For this review, take the finished solid that the model builds, in its own axes (mm). Give positions to 0.01 mm unless a question says otherwise; leave off trailing zeros. Order: outer loops, then holes, each group sorted by start corner. A loop starts at its lowest first (then second) coordinate and runs counter-clockwise, first axis right, second up. Notation, with made-up numbers: (24, -7) -> (39, -7) arc R31 cw to (39, 17) -> close; hole circle Ø2 at (-0.5, 40). An arc over 180 degrees is marked (long way). Return JSON: item names as keys, results as strings. Group by question number.
1) Add section D-D (z = -6). Give the boundary of the cut face in (x, y).
2) Insertion check: P1, Ø0.7, axis at x = 27, y = 2, coming from the -Z side; P2, Ø1.5, axis at y = 2, z = -51.5, coming from the -X side; P3, Ø2.5, axis at x = 14, z = -5.2, coming from the -Y side. Each pin has a flat end and moves straight along its axis. Give the tip position at first contact, or say it passes through.
3) To check wall thickness, follow line 1 along X through (y, z) = (1.45, -36.2); line 2 along Z through (x, y) = (14, 2.05); line 3 along Z through (x, y) = (54.1, 1.15). State the ranges of each line that lie inside material, in increasing order.
4) Add section C-C (x = 45). Give the boundary of the cut face in (y, z), then the cut area to 3 significant figures.
5) Add section B-B (z = -42). Give the boundary of the cut face in (x, y), then the cut area to 3 significant figures.
6) Add section A-A (x = 29.5). Give the boundary of the cut face in (y, z).
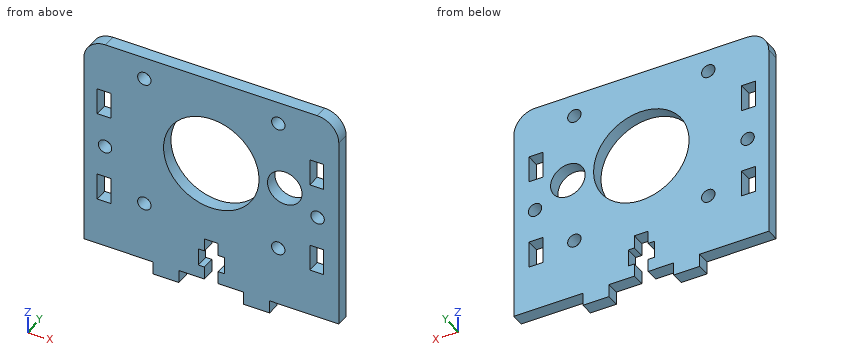
from build123d import *

# Parameters (mm, degrees)
CROQUIS1_R              = 1.55
CROQUIS1_R_2            = 11.05
CROQUIS1_R_3            = 4
CROQUIS1_W              = 3.2
CROQUIS1_H              = 6.2
SALIENTE_EXTRUIR1_DEPTH = 3


with BuildPart() as part:
    # Croquis1 → Saliente-Extruir1 (new body)
    with BuildSketch(Plane(origin=(0, 0, 0), x_dir=(1, 0, 0), z_dir=(0, 1, 0))):
        with BuildLine():
            Line((5, 0), (54, 0))
            ThreePointArc((54, 0), (57.535533906, 1.464466094), (59, 5))
            Line((59, 5), (59, 50))
            Line((59, 50), (43, 50))
            Line((43, 50), (43, 53))
            Line((43, 53), (37, 53))
            Line((37, 53), (37, 50))
            Line((37, 50), (31.1, 50))
            Line((31.1, 50), (31.1, 47))
            Line((31.1, 47), (32.5, 47))
            Line((32.5, 47), (32.5, 43))
            Line((32.5, 43), (31.1, 43))
            Line((31.1, 43), (31.1, 40))
            Line((31.1, 40), (27.9, 40))
            Line((27.9, 40), (27.9, 43))
            Line((27.9, 43), (26.5, 43))
            Line((26.5, 43), (26.5, 47))
            Line((26.5, 47), (27.9, 47))
            Line((27.9, 47), (27.9, 50))
            Line((27.9, 50), (22, 50))
            Line((22, 50), (22, 53))
            Line((22, 53), (16, 53))
            Line((16, 53), (16, 50))
            Line((16, 50), (0, 50))
            Line((0, 50), (0, 5))
            ThreePointArc((0, 5), (1.464466094, 1.464466094), (5, 0))
        make_face()
        with Locations((4.9, 25.3)):
            Circle(CROQUIS1_R, mode=Mode.SUBTRACT)
        with Locations((29.5, 20.7)):
            Circle(CROQUIS1_R_2, mode=Mode.SUBTRACT)
        with Locations((14, 36.2)):
            Circle(CROQUIS1_R, mode=Mode.SUBTRACT)
        with Locations((45, 36.2)):
            Circle(CROQUIS1_R, mode=Mode.SUBTRACT)
        with Locations((45, 5.2)):
            Circle(CROQUIS1_R, mode=Mode.SUBTRACT)
        with Locations((14, 5.2)):
            Circle(CROQUIS1_R, mode=Mode.SUBTRACT)
        with Locations((46.5, 20.7)):
            Circle(CROQUIS1_R_3, mode=Mode.SUBTRACT)
        with Locations((54.1, 25.3)):
            Circle(CROQUIS1_R, mode=Mode.SUBTRACT)
        with Locations((4.7, 14.7)):
            Rectangle(CROQUIS1_W, CROQUIS1_H, mode=Mode.SUBTRACT)
        with Locations((4.7, 35.9)):
            Rectangle(CROQUIS1_W, CROQUIS1_H, mode=Mode.SUBTRACT)
        with Locations((53.9, 35.9)):
            Rectangle(CROQUIS1_W, CROQUIS1_H, mode=Mode.SUBTRACT)
        with Locations((53.9, 14.7)):
            Rectangle(CROQUIS1_W, CROQUIS1_H, mode=Mode.SUBTRACT)
    extrude(amount=SALIENTE_EXTRUIR1_DEPTH)


solid = part.part
Evaluation:
{
 "1": {"outline": "(0, 0) -> (12.67, 0) -> (12.67, 3) -> (0, 3) -> close; (15.33, 0) -> (43.67, 0) -> (43.67, 3) -> (15.33, 3) -> close; (46.33, 0) -> (59, 0) -> (59, 3) -> (46.33, 3) -> close"},
 "2": {"P1": "z = -50", "P2": "x = 16", "P3": "through"},
 "3": {"line 1": "0 to 3.1, 6.3 to 12.45, 15.55 to 43.45, 46.55 to 52.3, 55.5 to 59", "line 2": "-50 to -37.75, -34.65 to -6.75, -3.65 to 0", "line 3": "-50 to -39, -32.8 to -26.85, -23.75 to -17.8, -11.6 to 0"},
 "4": {"outline": "(0, -50) -> (3, -50) -> (3, -37.75) -> (0, -37.75) -> close; (0, -34.65) -> (3, -34.65) -> (3, -24.41) -> (0, -24.41) -> close; (0, -16.99) -> (3, -16.99) -> (3, -6.75) -> (0, -6.75) -> close; (0, -3.65) -> (3, -3.65) -> (3, 0) -> (0, 0) -> close", "area": "109 mm^2"},
 "5": {"outline": "(0, 0) -> (27.9, 0) -> (27.9, 3) -> (0, 3) -> close; (31.1, 0) -> (59, 0) -> (59, 3) -> (31.1, 3) -> close", "area": "167 mm^2"},
 "6": {"outline": "(0, -40) -> (3, -40) -> (3, -31.75) -> (0, -31.75) -> close; (0, -9.65) -> (3, -9.65) -> (3, 0) -> (0, 0) -> close"}
}
